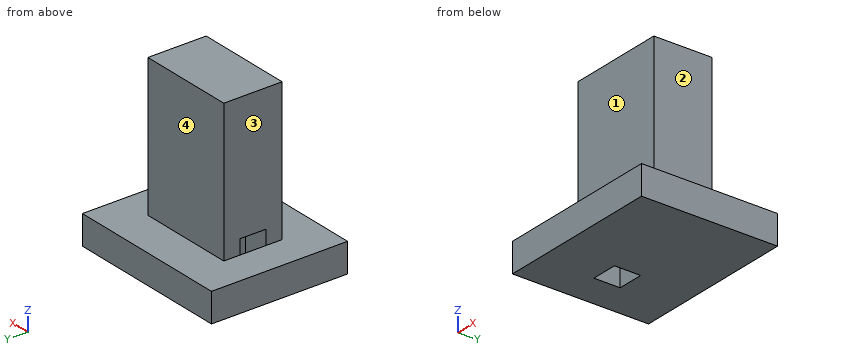
from build123d import *

# Parameters (mm, degrees)
SKETCH1_W           = 8.5
SKETCH1_H           = 7
SKETCH1_W_2         = 5
SKETCH1_H_2         = 3
BOSS_EXTRUDE1_DEPTH = 1.5
BOSS_EXTRUDE2_DEPTH = 2.25
SKETCH3_W           = 5
SKETCH3_H           = 3
BOSS_EXTRUDE3_DEPTH = 6.5


with BuildPart() as part:
    # Sketch1 → Boss-Extrude1 (new body)
    with BuildSketch(Plane.XY):
        with Locations((2.5, 1.5)):
            Rectangle(SKETCH1_W, SKETCH1_H)
        with Locations((2.5, 1.5)):
            Rectangle(SKETCH1_W_2, SKETCH1_H_2, mode=Mode.SUBTRACT)
    extrude(amount=BOSS_EXTRUDE1_DEPTH)

    # Sketch1_3 → Boss-Extrude2 (add)
    with BuildSketch(Plane.XY):
        Polygon((0, 0.825), (0, 0), (5, 0), (5, 3), (0, 3), (0, 2.175), (1.35, 2.175), (1.35, 0.825), align=None)
    extrude(amount=BOSS_EXTRUDE2_DEPTH)

    # Sketch3 → Boss-Extrude3 (add)
    with BuildSketch(Plane.XY.offset(2.25)):
        with Locations((2.5, 1.5)):
            Rectangle(SKETCH3_W, SKETCH3_H)
    extrude(amount=BOSS_EXTRUDE3_DEPTH)


solid = part.part
Can you work these out from the model? Positions are in its coordinate system, mm. Face numbers are marked on the shaded views. A direction names the side the tool comes from. Round coordinates to 2 decimals unless told otherwise and drop trailing zeros. Order: outer loops, then holes, each group sorted by start corner. A loop starts at its lowest first (then second) coordinate and runs counter-clockwise, first axis right, second up. Notation, with made-up numbers: (83, 32) - (118, 32) arc R26 cw to (118, 48) - close; hole circle Ø5 at (-30.5, 42). An arc over 180 degrees is marked (long way). Answer in a Markdown table with one row per item.
(1) For P1, Ø1, axis at y = -1, z = 6, coming from the +X side; P2, Ø3.5, axis at y = 2, z = 5.5, coming from the +X side; P3, Ø3, axis at x = 5, z = 3.5, coming from the -Y side; P4, Ø5, axis at x = 3.5, z = 5.5, coming from the +Y side, each with a flat end and sliding along its axis, tell me the tip position at first contact or that it passes through.
From the geometry:
| item | result |
|---|---|
| P1 | passes through |
| P2 | stops at x = 5 |
| P3 | stops at y = 0 |
| P4 | stops at y = 3 |
(2) Suppose I cut it at B-B, the plane x = 1.75. Please give me the cut outline in (y, z), plus the area to 4 significant figures.
From the geometry:
| item | result |
|---|---|
| outline | (-2, 0) - (5, 0) - (5, 1.5) - (3, 1.5) - (3, 8.75) - (0, 8.75) - (0, 1.5) - (-2, 1.5) - close |
| area | 32.25 mm2 |
(3) Please list where these lines run through material, in increasing order: L1, parallel to X at y = 1, z = 0.5; L2, parallel to Y at x = 1.75, z = 3.5; L3, parallel to Z at x = 3.25, y = 4.75. Write a range as from..to.
From the geometry:
| item | result |
|---|---|
| L1 | x = -1.75..0, 1.35..6.75 |
| L2 | y = 0..3 |
| L3 | z = 0..1.5 |
(4) Suppose I cut it at D-D, the plane z = 3. Please give me the cut outline in (x, y), plus the area to 3 significant figures.
From the geometry:
| item | result |
|---|---|
| outline | (0, 0) - (5, 0) - (5, 3) - (0, 3) - close |
| area | 15.0 mm2 |
(5) Suppose I cut it at A-A, the plane z = 1. Please give me the cut outline in (x, y) (3 decimals), plus the area to 3 significant figures.
From the geometry:
| item | result |
|---|---|
| outline | (-1.75, -2) - (6.75, -2) - (6.75, 5) - (-1.75, 5) - close; hole (0, 0.825) - (1.35, 0.825) - (1.35, 2.175) - (0, 2.175) - close |
| area | 57.7 mm2 |
(6) Which directions (+Z, -Z, +X, -X, +Y, -Y) give clear straight access to the entire face, cutting with the end or side of a thin tool? Please do the marked faces 1, 2, 3 and 4.
From the geometry:
| item | result |
|---|---|
| face 1 | +Z, +X, -X, -Y |
| face 2 | +Z, +X, +Y, -Y |
| face 3 | +Z, -X, +Y, -Y |
| face 4 | +Z, +X, -X, +Y |
(7) Suppose I cut it at C-C, the plane y = 0.5. Please give me the cut outline in (x, z).
From the geometry:
| item | result |
|---|---|
| outline | (-1.75, 0) - (6.75, 0) - (6.75, 1.5) - (5, 1.5) - (5, 8.75) - (0, 8.75) - (0, 1.5) - (-1.75, 1.5) - close |
